Here's how the part is built. I have some questions about the finished solid (model axes, mm). A direction names the side the tool comes from. Give positions to 0.01 mm unless a question says otherwise; leave off trailing zeros. Loops run counter-clockwise (first coordinate to the right, second up) from the corner with the lowest first, then second, coordinate; pieces in that order, holes last. Notation, with made-up numbers: (88.5, -37.5) - (108.5, -37.5) arc R21 cw to (108.5, -12.5) - close; hole circle Ø2 at (10.25, -31). An arc over 180 degrees is marked (long way). Use a Markdown table: item, result.
from build123d import *

# Parameters (mm, degrees)
SKETCH1_W                      = 114.3
SKETCH1_H                      = 114.3
SEEBECK_MIDDLE_BLOCK_DEPTH     = 9.525
SKETCH2_R                      = 0.79375
THERMO_COUPLE_HOLE_DEPTH       = 60.325
SKETCH3_R                      = 4.7625
MIDDLE_MOUNTING_HOLES_DEPTH    = 116.31336133
F_9_0_196_TEG_MOUNT_HOLE_D     = 4.9784
F_9_0_196_TEG_MOUNT_HOLE_DEPTH = 6.35
F_9_0_196_TEG_MOUNT_HOLE_TIP   = 1.495662253
F_9_0_196_VOLTAGE_HOLE_D       = 4.9784
F_9_0_196_VOLTAGE_HOLE_DEPTH   = 12.7
F_9_0_196_VOLTAGE_HOLE_TIP     = 1.495662253


with BuildPart() as part:
    # Sketch1 → Seebeck Middle Block (new body)
    with BuildSketch(Plane(origin=(0, 0, 0), x_dir=(1, 0, 0), z_dir=(0, 1, 0))):
        with Locations((24.209375, -24.0109375)):
            Rectangle(SKETCH1_W, SKETCH1_H)
    extrude(amount=SEEBECK_MIDDLE_BLOCK_DEPTH)

    # Sketch2 → Thermo Couple Hole (cut)
    with BuildSketch(Plane.ZY.offset(32.940625)):
        with Locations((24.0109375, 3.175)):
            Circle(SKETCH2_R)
    extrude(amount=-THERMO_COUPLE_HOLE_DEPTH, mode=Mode.SUBTRACT)

    # Sketch3 → Middle Mounting holes (cut, through all)
    with BuildSketch(Plane(origin=(0, 9.525, 0), x_dir=(1, 0, 0), z_dir=(0, 1, 0))):
        with Locations(Location((-25.796875, -55.7609375, 0), (0, 0, 270))):
            Circle(SKETCH3_R)
        with Locations(Location((-25.796875, 7.7390625, 0), (0, 0, 270))):
            Circle(SKETCH3_R)
        with Locations(Location((72.628125, -24.0109375, 0), (0, 0, 270))):
            Circle(SKETCH3_R)
    extrude(amount=-MIDDLE_MOUNTING_HOLES_DEPTH, mode=Mode.SUBTRACT)

    # #9 (0.196) TEG Mount Hole
    with Locations(Plane(origin=(0, 9.525, 0), x_dir=(1, 0, 0), z_dir=(0, 1, 0))):
        with Locations((-4.365625, 4.5640625), (54.371875, 4.5640625), (54.371875, -54.1734375), (-4.365625, -54.1734375)):
            Hole(F_9_0_196_TEG_MOUNT_HOLE_D / 2, depth=F_9_0_196_TEG_MOUNT_HOLE_DEPTH)
            with Locations((0, 0, -(F_9_0_196_TEG_MOUNT_HOLE_DEPTH + F_9_0_196_TEG_MOUNT_HOLE_TIP / 2))):  # 118° drill point
                Cone(0, F_9_0_196_TEG_MOUNT_HOLE_D / 2, F_9_0_196_TEG_MOUNT_HOLE_TIP, mode=Mode.SUBTRACT)

    # #9 (0.196) Voltage Hole
    with Locations(Plane(origin=(81.359375, 0, 0), x_dir=(0, 0, -1), z_dir=(1, 0, 0))):
        with Locations((-38.827604082, 4.7625)):
            Hole(F_9_0_196_VOLTAGE_HOLE_D / 2, depth=F_9_0_196_VOLTAGE_HOLE_DEPTH)
            with Locations((0, 0, -(F_9_0_196_VOLTAGE_HOLE_DEPTH + F_9_0_196_VOLTAGE_HOLE_TIP / 2))):  # 118° drill point
                Cone(0, F_9_0_196_VOLTAGE_HOLE_D / 2, F_9_0_196_VOLTAGE_HOLE_TIP, mode=Mode.SUBTRACT)


solid = part.part
(1) If I drill on line 1 (Z direction, x = -4.5, y = 3.5); line 2 (Z direction, x = 9.5, y = 2.5); line 3 (Z direction, x = 23, y = 3.5), over which ranges is the centre line in solid material (lowest first)?
A:
| item | result |
|---|---|
| line 1 | -33.14 to -7.05, -2.08 to 23.29, 24.74 to 51.69, 56.66 to 81.16 |
| line 2 | -33.14 to 23.59, 24.43 to 81.16 |
| line 3 | -33.14 to 23.29, 24.74 to 81.16 |
(2) On a 3-axis mill with a long thin cutter (end or side, diameter ignored), from which of +Z, -Z, +X, -X, +Y, -Y can I reach the whole of each face in a straight line? I mean faces 5 (the face through (23, 9.525, 23)), 6 (the face through (74.92, 3.809, 41.127)), 7 (the face through (-5.704, 6.306, -6.663)). Say none if no direction works.
A:
| item | result |
|---|---|
| face 5 | +Z, -Z, +X, -X, +Y |
| face 6 | +X |
| face 7 | +Y |
(3) Will these pins go through, and if not, where does the flat tip stop? pin 1 (6.5 mm diameter, centred on x = -4.37, z = 54.17, fed in from -Y); pin 2 (3 mm diameter, centred on y = 4.76, z = 38.83, fed in from +X); pin 3 (5.5 mm diameter, centred on x = 72.63, z = 24.01, fed in from +Y); pin 4 (0.8 mm diameter, centred on y = 3.5, z = 24, fed in from -X).
A:
| item | result |
|---|---|
| pin 1 | y = 0 |
| pin 2 | x = 68.07 |
| pin 3 | through |
| pin 4 | x = 27.38 |
(4) Suppose I cut it at A-A on x = 71. Write out the boundary of the cut face in (y, z) (1 decimal), plus the area to 3 significant figures.
A:
| item | result |
|---|---|
| outline | (0, -33.1) - (9.5, -33.1) - (9.5, 19.5) - (0, 19.5) - close; (0, 28.5) - (9.5, 28.5) - (9.5, 81.2) - (0, 81.2) - close; hole circle Ø5 at (4.8, 38.8) |
| area | 984 mm2 |
(5) We'd pull the mould along Z, two halves only. Please class faces 1 (the face through (81.359, 5, 25)), 2 (the face through (52.072, 6.306, 55.127)), 3 (the face through (23, 5, 81.161)), 4 (the face through (-28.69, 4.83, 51.98)): pulls with the +Z half, pulls with the -Z half, needs draft (parallel to the pull), parting line crosses it, or undercut.
A:
| item | result |
|---|---|
| face 1 | needs draft |
| face 2 | undercut |
| face 3 | pulls with the +Z half |
| face 4 | undercut |
